Verification items for this drawing (mm, ordinates from the low corner). Round coordinates to 2 decimals unless told otherwise and drop trailing zeros. Order: outer loops, then holes, each group sorted by start corner. A loop starts at its lowest first (then second) coordinate and runs counter-clockwise, first axis right, second up. Notation, with made-up numbers: (40, -5.75) -> (68, -5.75) arc R11 ccw to (68, 2.25) -> close; hole circle Ø9 at (55.25, 6.25). An arc over 180 degrees is marked (long way). Answer in a Markdown table with one row per item. Add a question column.
1. Material ranges on L1, parallel to Z at x = 2.4, y = 1; L2, parallel to Z at x = 3.2, y = 3.1; L3, parallel to X at y = 0.2, z = 14.5, recorded low to high. Write a range as from..to.
2. Sectioned sample at C-C, the plane z = 1.5. Record the boundary of the cut face in (x, y), then the cut area to 3 significant figures.
3. Sectioned sample at B-B, the plane x = 0.65. Record the boundary of the cut face in (y, z), then the cut area to 3 significant figures.
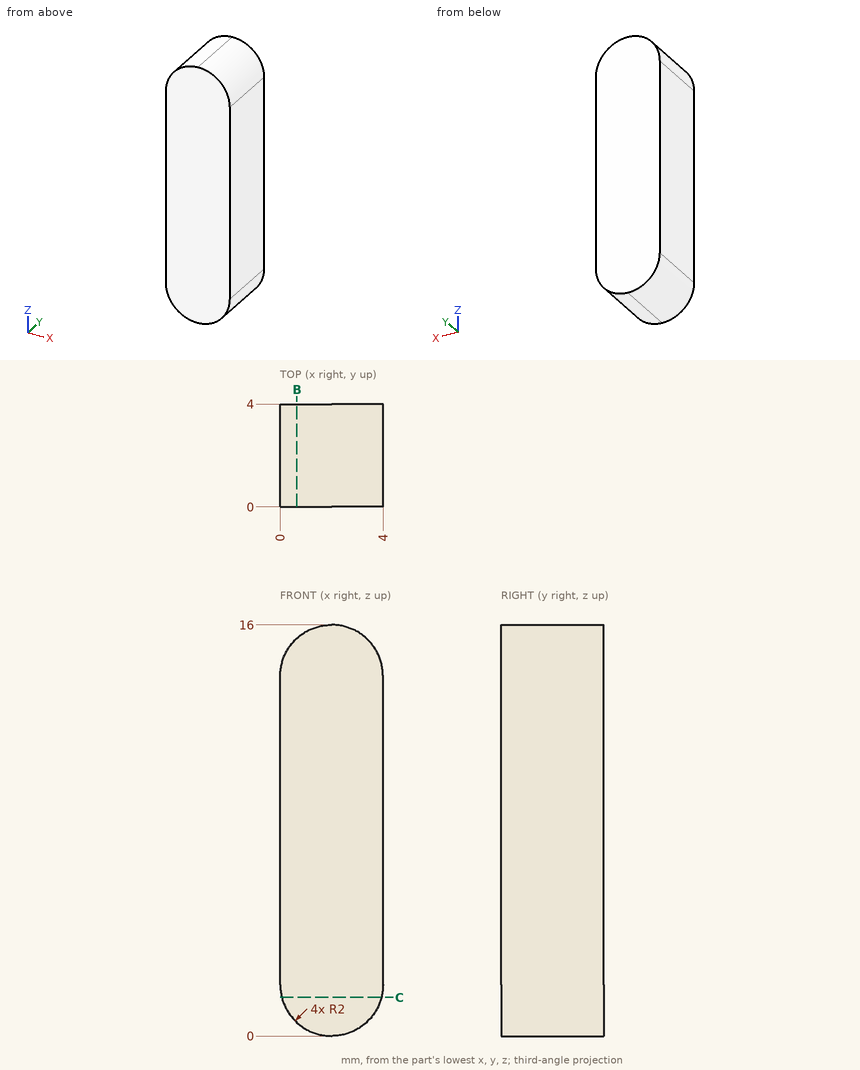
Answer key:
| question | item | result |
|---|---|---|
| 1 | L1 | z = 0.04..15.96 |
| 1 | L2 | z = 0.4..15.6 |
| 1 | L3 | x = 0.06..3.94 |
| 2 | outline | (0.06, 0) -> (3.94, 0) -> (3.94, 4) -> (0.06, 4) -> close |
| 2 | area | 15.5 mm² |
| 3 | outline | (0, 0.52) -> (4, 0.52) -> (4, 15.48) -> (0, 15.48) -> close |
| 3 | area | 59.8 mm² |
